Design review of the part built by this model. Coordinates are the model's own, in mm. A direction names the side the tool comes from. Coordinates: 2 decimals unless noted, no trailing zeros. Order: outer loops, then holes, each group sorted by start corner. A loop starts at its lowest first (then second) coordinate and runs counter-clockwise, first axis right, second up.
from build123d import *

# Parameters (mm, degrees)
F0_R     = 2.95
F0_R_2   = 2.575
F1_DEPTH = 0.8
F0_R_3   = 2.45
F2_DEPTH = 0.8
F0_R_4   = 1.65
F3_DEPTH = 7.8
F4_DEPTH = 7.8
F5_DEPTH = 7.1
F6_DEPTH = 7.8
F7_DEPTH = 0.8


# Not quite as in the source:
# - a fillet or chamfer that OpenCascade refuses, or shapes differently, is made with other operations: its cross-section is extruded or revolved along the edge and cut away or added


with BuildPart() as f1:
    # F0 (on Front) → F1 (new body)
    with BuildSketch(Plane.XZ):
        with Locations((-40.3700359166, 25.8709397167)):
            Circle(F0_R)
        with Locations((-40.3700359166, 25.8709397167)):
            Circle(F0_R_2, mode=Mode.SUBTRACT)
    extrude(amount=F1_DEPTH)

    # F0 (on Front) → F2 (join)
    with BuildSketch(Plane.XZ):
        with Locations((-40.3700359166, 25.8709397167)):
            Circle(F0_R_2)
        with Locations((-40.3700359166, 25.8709397167)):
            Circle(F0_R_3, mode=Mode.SUBTRACT)
    extrude(amount=F2_DEPTH)

    # F0 (on Front) → F3 (join)
    with BuildSketch(Plane.XZ):
        with Locations((-40.3700359166, 25.8709397167)):
            Circle(F0_R_3)
        with Locations((-40.3700359166, 25.8709397167)):
            Circle(F0_R_4, mode=Mode.SUBTRACT)
    extrude(amount=F3_DEPTH)

    # F0 (on Front) → F4 (join)
    with BuildSketch(Plane.XZ):
        with Locations((-40.3700359166, 25.8709397167)):
            Circle(F0_R_2)
        with Locations((-40.3700359166, 25.8709397167)):
            Circle(F0_R_3, mode=Mode.SUBTRACT)
    extrude(amount=F4_DEPTH)

    # F0 (on Front) → F5 (cut)
    with BuildSketch(Plane.XZ):
        with Locations((-40.3700359166, 25.8709397167)):
            Circle(F0_R_2)
        with Locations((-40.3700359166, 25.8709397167)):
            Circle(F0_R_3, mode=Mode.SUBTRACT)
    extrude(amount=F5_DEPTH, mode=Mode.SUBTRACT)

    # F0 (on Front) → F6 (join)
    with BuildSketch(Plane.XZ):
        with Locations((-40.3700359166, 25.8709397167)):
            Circle(F0_R_3)
        with Locations((-40.3700359166, 25.8709397167)):
            Circle(F0_R_4, mode=Mode.SUBTRACT)
    extrude(amount=-F6_DEPTH)

    # F0 (on Front) → F7 (join)
    with BuildSketch(Plane.XZ):
        with Locations((-40.3700359166, 25.8709397167)):
            Circle(F0_R)
        with Locations((-40.3700359166, 25.8709397167)):
            Circle(F0_R_2, mode=Mode.SUBTRACT)
        with Locations((-40.3700359166, 25.8709397167)):
            Circle(F0_R_2)
        with Locations((-40.3700359166, 25.8709397167)):
            Circle(F0_R_3, mode=Mode.SUBTRACT)
    extrude(amount=-F7_DEPTH)

    # F8: F1 across plane


with BuildPart() as f1_1:
    add(f1.part)
    add(f1.part.mirror(Plane.XZ))

    # F9: fillet of radius 0.2 on 6 edges, made by hand

    # F9_s1 → F9_t2 (revolve, cut)
    with BuildSketch(Plane.XY.offset(25.8709397167)):
        with BuildLine():
            ThreePointArc((-38.5190702311, -7.8004), (-38.6614572728, -7.7414213562), (-38.7204359166, -7.5990343146))
            Line((-38.7204359166, -7.5990343146), (-38.7405724851, -7.5990343146))
            ThreePointArc((-38.7405724851, -7.5990343146), (-38.7401724851, -7.6995171573), (-38.7401724851, -7.8))
            Line((-38.7401724851, -7.8), (-38.7200359166, -7.8201365685))
            ThreePointArc((-38.7200359166, -7.8201365685), (-38.6195530739, -7.8201365685), (-38.5190702311, -7.8205365685))
            Line((-38.5190702311, -7.8205365685), (-38.5190702311, -7.8004))
        make_face()
    revolve(axis=Axis((-40.3700359166, -7.8, 25.8709397167), (0, -1, 0)), mode=Mode.SUBTRACT)

    # F9_s3 → F9_t4 (revolve, cut)
    with BuildSketch(Plane.XY.offset(25.8709397167)):
        with BuildLine():
            ThreePointArc((-37.7946359166, -7.5990343146), (-37.8536145603, -7.7414213562), (-37.996001602, -7.8004))
            Line((-37.996001602, -7.8004), (-37.996001602, -7.8205365685))
            ThreePointArc((-37.996001602, -7.8205365685), (-37.8955187593, -7.8201365685), (-37.7950359166, -7.8201365685))
            Line((-37.7950359166, -7.8201365685), (-37.774899348, -7.8))
            ThreePointArc((-37.774899348, -7.8), (-37.774899348, -7.6995171573), (-37.774499348, -7.5990343146))
            Line((-37.774499348, -7.5990343146), (-37.7946359166, -7.5990343146))
        make_face()
    revolve(axis=Axis((-40.3700359166, -7.8, 25.8709397167), (0, -1, 0)), mode=Mode.SUBTRACT)

    # F9_s5 → F9_t6 (revolve, cut)
    with BuildSketch(Plane.XY.offset(25.8709397167)):
        with BuildLine():
            ThreePointArc((-37.9198847153, -7.0996296783), (-37.828855755, -7.173758828), (-37.7946359166, -7.286054888))
            Line((-37.7946359166, -7.286054888), (-37.774499348, -7.286054888))
            ThreePointArc((-37.774499348, -7.286054888), (-37.774899348, -7.193027444), (-37.774899348, -7.1))
            Line((-37.774899348, -7.1), (-37.7950359166, -7.0798634315))
            ThreePointArc((-37.7950359166, -7.0798634315), (-37.8574603159, -7.0798634315), (-37.9122730266, -7.0809871573))
            Line((-37.9122730266, -7.0809871573), (-37.9198847153, -7.0996296783))
        make_face()
    revolve(axis=Axis((-40.3700359166, -7.1, 25.8709397167), (0, -1, 0)), mode=Mode.SUBTRACT)

    # F9_s7 → F9_t8 (revolve, cut)
    with BuildSketch(Plane.XY.offset(25.8709397167)):
        with BuildLine():
            ThreePointArc((-37.996001602, 7.8004), (-37.8536145603, 7.7414213562), (-37.7946359166, 7.5990343146))
            Line((-37.7946359166, 7.5990343146), (-37.774499348, 7.5990343146))
            ThreePointArc((-37.774499348, 7.5990343146), (-37.774899348, 7.6995171573), (-37.774899348, 7.8))
            Line((-37.774899348, 7.8), (-37.7950359166, 7.8201365685))
            ThreePointArc((-37.7950359166, 7.8201365685), (-37.8955187593, 7.8201365685), (-37.996001602, 7.8205365685))
            Line((-37.996001602, 7.8205365685), (-37.996001602, 7.8004))
        make_face()
    revolve(axis=Axis((-40.3700359166, 7.8, 25.8709397167), (0, -1, 0)), mode=Mode.SUBTRACT)

    # F9_s9 → F9_t10 (revolve, cut)
    with BuildSketch(Plane.XY.offset(25.8709397167)):
        with BuildLine():
            ThreePointArc((-37.9198847153, 7.0996296783), (-37.828855755, 7.173758828), (-37.7946359166, 7.286054888))
            Line((-37.7946359166, 7.286054888), (-37.774499348, 7.286054888))
            ThreePointArc((-37.774499348, 7.286054888), (-37.774899348, 7.193027444), (-37.774899348, 7.1))
            Line((-37.774899348, 7.1), (-37.7950359166, 7.0798634315))
            ThreePointArc((-37.7950359166, 7.0798634315), (-37.8574603159, 7.0798634315), (-37.9122730266, 7.0809871573))
            Line((-37.9122730266, 7.0809871573), (-37.9198847153, 7.0996296783))
        make_face()
    revolve(axis=Axis((-40.3700359166, 7.1, 25.8709397167), (0, -1, 0)), mode=Mode.SUBTRACT)

    # F9_s11 → F9_t12 (revolve, cut)
    with BuildSketch(Plane.XY.offset(25.8709397167)):
        with BuildLine():
            ThreePointArc((-38.7204359166, 7.5990343146), (-38.6614572728, 7.7414213562), (-38.5190702311, 7.8004))
            Line((-38.5190702311, 7.8004), (-38.5190702311, 7.8205365685))
            ThreePointArc((-38.5190702311, 7.8205365685), (-38.6195530739, 7.8201365685), (-38.7200359166, 7.8201365685))
            Line((-38.7200359166, 7.8201365685), (-38.7401724851, 7.8))
            ThreePointArc((-38.7401724851, 7.8), (-38.7401724851, 7.6995171573), (-38.7405724851, 7.5990343146))
            Line((-38.7405724851, 7.5990343146), (-38.7204359166, 7.5990343146))
        make_face()
    revolve(axis=Axis((-40.3700359166, 7.8, 25.8709397167), (0, -1, 0)), mode=Mode.SUBTRACT)


solid = f1_1.part
1. Mouldability with a two-part tool opening along Y and no side actions: class faces 5 (the cylindrical face through (-39.053, 3.906, 27.937)), 6 (the flat face through (-42, -0.8, 28)), 7 (the cylindrical face through (-42.711, -0.011, 24.076)) as pulls with the +Y half, pulls with the -Y half, needs draft (parallel to the pull), parting line crosses it, or undercut.
2. Insertion check: pin 1 (2 mm diameter, centred on y = 3.5, z = 25, fed in from +X); pin 2 (2 mm diameter, centred on x = -40.37, z = 25.87, fed in from -Y). Each pin has a flat end and moves straight along its axis. Give the tip position at first contact, or say it passes through.
3. To check wall thickness, follow line 1 (Y direction, x = -39.3, z = 27.35); line 2 (Z direction, x = -40.85, y = -0.75); line 3 (Z direction, x = -39.8, y = -6.25). State the ranges of each line that lie inside material, in increasing order.
4. Add section A-A (y = 5.75). Give the boundary of the cut face in (x, z).
5. For faces 1 (the cylindrical face through (-40.73, 0.11, 24.26)), 2 (the cylindrical face through (-39.182, 7.44, 23.586)), 3 (the flat face through (-42, 0.8, 28)), 4 (the cylindrical face through (-39.182, -7.44, 23.586)), list the 3-axis set-ups (+Z, -Z, +X, -X, +Y, -Y) from which the entire face can be reached by the end or side of a thin tool; tool diameter is ignored.
Solution:
1. face 5: undercut
1. face 6: undercut
1. face 7: needs draft
2. pin 1: stops at x = -37.92
2. pin 2: passes through
3. line 1: y = -7.8 to 7.8
3. line 2: z = 22.96 to 24.29, 27.45 to 28.78
3. line 3: z = 23.49 to 24.32, 27.42 to 28.25
4. outline: circle Ø4.9 at (-40.37, 25.87); hole circle Ø3.3 at (-40.37, 25.87)
5. face 1: +Y, -Y
5. face 2: +Y
5. face 3: none
5. face 4: -Y
